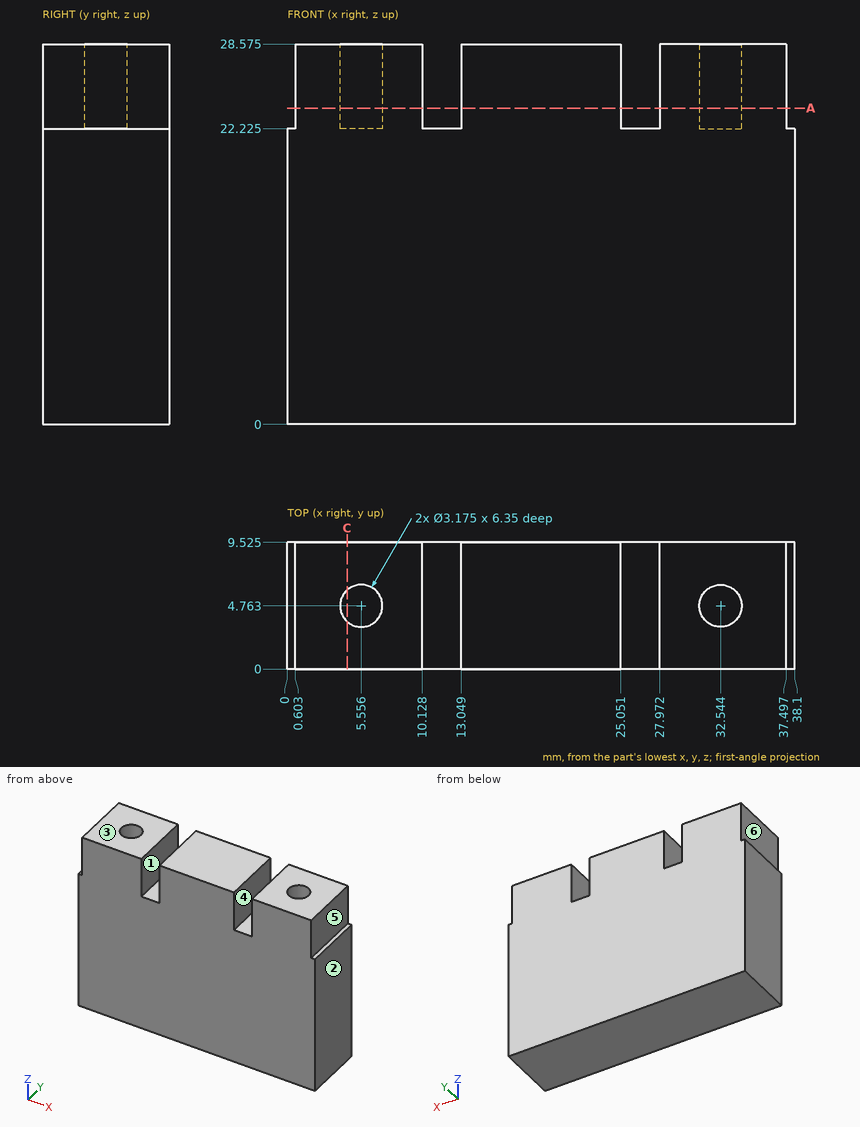
The drawing under review shows one solid part. Ordinate dimensions are in mm from its lowest x, y, z. A direction names the side the tool comes from. Give positions to 0.01 mm unless a question says otherwise; leave off trailing zeros. Write each loop counter-clockwise with the first axis right and the second up, starting at its lowest first coordinate (ties: lowest second). Pieces come first, ordered by that corner, then holes. Notation, with made-up numbers: (28.5, 46.5) -> (66.5, 46.5) arc R17 cw to (66.5, 54.5) -> close; hole circle Ø6 at (12, 14.25). An arc over 180 degrees is marked (long way). Answer in a Markdown table with one row per item.
(1) For the marked faces 4, 5 and 6, list the 3-axis set-ups (+Z, -Z, +X, -X, +Y, -Y) from which the entire face can be reached by the end or side of a thin tool; tool diameter is ignored.
Results:
| item | result |
|---|---|
| face 4 | +Z, +Y, -Y |
| face 5 | +Z, +X, +Y, -Y |
| face 6 | +Z, -X, +Y, -Y |
(2) Mouldability with a two-part tool opening along X and no side actions: class the marked faces 1, 2 and 3 as +X half, -X half, draft (parallel to the pull), parting line (faces both ways), or undercut.
Results:
| item | result |
|---|---|
| face 1 | undercut |
| face 2 | +X half |
| face 3 | draft |
(3) Consider section C-C (x = 4.5). State the section outline as (y, z) points (1 decimal), then the cut area to 3 significant figures.
Results:
| item | result |
|---|---|
| outline | (0, 0) -> (9.5, 0) -> (9.5, 28.6) -> (5.9, 28.6) -> (5.9, 22.2) -> (3.6, 22.2) -> (3.6, 28.6) -> (0, 28.6) -> close |
| area | 257 mm2 |
(4) To check wall thickness, follow probe 1 along X at (y, z) = (3, 22.5); probe 2 along Z at (x, y) = (10.5, 3.75) (1 decimal). State the ranges of each line that lie inside material, in increasing order.
Results:
| item | result |
|---|---|
| probe 1 | 0.6 to 10.13, 13.05 to 25.05, 27.97 to 37.5 |
| probe 2 | 0 to 22.2 |
(5) Clearance check with flat-ended pins moving along their axes: pin 1 (0.9 mm diameter, centred on x = 12, y = 4.5, fed in from +Z) (1 decimal); pin 2 (1.9 mm diameter, centred on y = 6, z = 24.5, fed in from +X); pin 3 (5 mm diameter, centred on y = 6, z = 26, fed in from -X). State where each tip first meets the part, or that it passes through.
Results:
| item | result |
|---|---|
| pin 1 | z = 22.2 |
| pin 2 | x = 37.5 |
| pin 3 | x = 0.6 |
(6) Consider section A-A (z = 23.75). Count the separate pieces of the cut face and the enclosed holes in it, then the cut area to 3 significant figures.
Results:
| item | result |
|---|---|
| separate pieces | 3 |
| enclosed holes | 2 |
| area | 280 mm2 |
